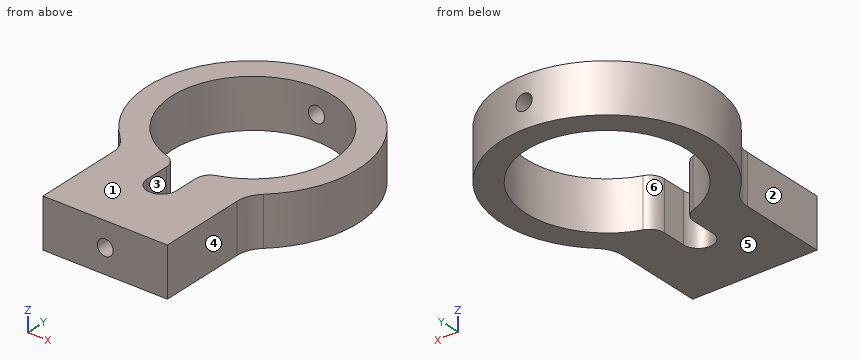
Autodesk Inventor part; units mm, degrees
ref_plane "Work Plane1" through (0, 21.5, 0) normal (0, 1, 0) x (-1, 0, 0)
ref_plane "Work Plane2" through (0, 0, 5) normal (0, 0, 1) x (1, 0, 0)
ref_plane "YZ Plane" through (0, 0, 0) normal (1, 0, 0) x (0, 1, 0)
sketch "Sketch1" plane through (0, 0, 0) normal (0, 0, 1) x (1, 0, 0)
  circle A0 centre (0, 0) radius 15 construction
  circle A1 centre (0, 0) radius 16.5
  circle A2 centre (0, 0) radius 21.5
  line L0 (0, 0) -> (26.2932, 0) construction
  line L1 (0, 0) -> (0, -21.5) construction
  line L2 (-12.7, -38.1) -> (12.7, -38.1)
  line L3 (12.7, -38.1) -> (12.7, -17.3482)
  line L4 (12.7, -17.3482) -> (-12.7, -17.3482)
  line L5 (-12.7, -17.3482) -> (-12.7, -38.1)
  line L6 (-12.7, -38.1) -> (12.7, -17.3482) construction
  line L7 (12.7, -38.1) -> (-12.7, -17.3482) construction
  point P0 (0, -27.7241)
  point P1 (0, -27.7241)
  dimension "d0" = 30
  dimension "d1" = 33
  dimension "d2" = 43
  dimension "d7" = 25.4
  dimension "d8" = 38.1
extrude "Extrusion1" add sketch "Sketch1" along normal blind 10
fillet "Fillet2" radius 6 2 edges at (12.7, -17.3482, 5) (-12.7, -17.3482, 5)
sketch "Sketch3" plane through (-12.7, -38.1, 0) normal (0, -1, 0) x (1, 0, 0)
  line L0 (0, 0) -> (0, 10)
  line L1 (12.7, 0) -> (12.7, 10) construction
  line L2 (-3.8, 10) -> (29.2, 10) construction
  line L3 (0, 5) -> (25.4, 5) construction
  line L4 (25.4, 10) -> (25.4, 0) construction
  point P0 (0.8561, 10)
  point P1 (24.5439, 10)
  point P2 (12.7, 5)
hole "Hole1" at (0, -38.1, 5) direction (0, 1, 0) diameter 3.242 depth 10 tip angle 118
ref_plane "Work Plane1" through (0, 21.5, 0) normal (0, 1, 0) x (-1, 0, 0)
sketch "Sketch4" plane through (0, 21.5, 0) normal (0, 1, 0) x (-1, 0, 0)
  line L0 (0, 0) -> (0, 10) construction
  line L1 (12.7, 10) -> (-12.7, 10) construction
  circle A0 centre (0, 5) radius 1.621 construction
  point P0 (0, 5)
hole "Hole2" at (0, 21.5, 5) direction (0, -1, 0) diameter 3.302 depth 12.3 tip angle 118
sketch "Sketch5" plane through (0, 0, 10) normal (0, 0, 1) x (1, 0, 0)
  circle A0 centre (0, 0) radius 16.5
  arc A1 (14.62, -15.7641) -> (-14.62, -15.7641) centre (0, 0) ccw
  line L0 (0, 0) -> (0, -38.1) construction
  line L1 (1.621, -38.1) -> (-1.621, -38.1) construction
  circle A2 centre (0, -23.5) radius 3
  line L2 (-3, -23.5) -> (-3, -16.225)
  line L3 (3, -23.5) -> (3, -16.225)
  line L4 (-12.7, -20.1633) -> (-12.7, -38.1)
  line L5 (12.7, -38.1) -> (12.7, -20.1633)
  line L6 (-12.7, -26.5) -> (12.7, -26.5) construction
  line L7 (12.7, -38.1) -> (12.7, -20.1633) construction
  line L8 (-10.4966, -16.5) -> (9.259, -16.5) construction
  dimension "d28" = 6
  dimension "d32" = 10
extrude "Extrusion3" cut sketch "Sketch5" against normal through all contours A0 L3 A2 L2 | A2
fillet "Fillet4" radius 3 2 edges at (-3, -16.225, 5) (3, -16.225, 5)
ref_plane "Work Plane2" through (0, 0, 5) normal (0, 0, 1) x (1, 0, 0)
properties part number "LaserTubeClamp"
Model file for the job. Use its own axes, mm. Face numbers are marked on the shaded views. A direction names the side the tool comes from. Round coordinates to 2 decimals unless told otherwise and drop trailing zeros. Write each loop counter-clockwise with the first axis right and the second up, starting at its lowest first coordinate (ties: lowest second). Pieces come first, ordered by that corner, then holes. Notation, with made-up numbers: (4.25, 89.5) - (9.25, 89.5) arc R21 ccw to (9.25, 105.5) - close; hole circle Ø2 at (70, -30). An arc over 180 degrees is marked (long way). Use CSV: the item, a comma, the result in double quotes. Start each with the question number.
Item 1: Band-saw the part on B-B (y = 0). Write the cut outline in (x, z), and give its area (3 significant figures).
Item 2: Drill centre lines: L1, parallel to Z at x = 0, y = -35.5; L2, parallel to Z at x = 0, y = 18; L3, parallel to Y at x = 0, z = 6.75. Where is each one in solid material? Low to high. Write a range as [from, to].
Item 3: Band-saw the part on C-C (x = -7.5). Write the cut outline in (y, z).
Item 4: Two-plate mould, pull along X, no slides. Class the marked faces 1, 2 and 3: released by +X, released by -X, zero draft, split by the parting line, or undercut.
Item 5: Pin check, flat tips, straight feed: P1, Ø5.5, axis at y = -21, z = 7, coming from the +X side; P2, Ø3, axis at y = -30, z = 6, coming from the +X side; P3, Ø5.5, axis at y = -22, z = 3, coming from the -X side. Stop position of each tip, or through.
Item 6: Tool access for the marked faces 4, 5 and 6: list every direction of +Z, -Z, +X, -X, +Y, -Y with a clear straight run to the whole face (end or side of a thin tool).
Item 7: Band-saw the part on A-A (z = 2.25). Write the cut outline in (x, y), and give its area (3 significant figures).
Checked values:
1,outline,"(-21.5, 0) - (-16.5, 0) - (-16.5, 10) - (-21.5, 10) - close; (16.5, 0) - (21.5, 0) - (21.5, 10) - (16.5, 10) - close"
1,area,"100 mm²"
2,L1,"z = [0, 3.38], [6.62, 10]"
2,L2,"z = [0, 3.35], [6.65, 10]"
2,L3,"y = [-38.1, -26.5], [16.5, 21.5]"
3,outline,"(-38.1, 0) - (-14.7, 0) - (-14.7, 10) - (-38.1, 10) - close; (14.7, 0) - (20.15, 0) - (20.15, 10) - (14.7, 10) - close"
4,face 1,"zero draft"
4,face 2,"released by -X"
4,face 3,"undercut"
5,P1,"stops at x = 13.01"
5,P2,"stops at x = 12.7"
5,P3,"stops at x = -12.77"
6,face 4,"+Z, -Z, +X, -Y"
6,face 5,"-Z, +X, -X, +Y, -Y"
6,face 6,"+Z, -Z"
7,outline,"(-14.62, -15.76) arc R6 cw to (-12.7, -20.16) - (-12.7, -38.1) - (12.7, -38.1) - (12.7, -20.16) arc R6 cw to (14.62, -15.76) arc R21.5 ccw (long way) to start; hole (-5.08, -15.7) arc R3 cw to (-3, -18.55) - (-3, -23.5) arc R3 ccw to (3, -23.5) - (3, -18.55) arc R3 cw to (5.08, -15.7) arc R16.5 ccw (long way) to start"
7,area,"996 mm²"
